Design review of the part built by this model. Coordinates are the model's own, in mm. A direction names the side the tool comes from. Give positions to 0.01 mm unless a question says otherwise; leave off trailing zeros. Loops run counter-clockwise (first coordinate to the right, second up) from the corner with the lowest first, then second, coordinate; pieces in that order, holes last. Notation, with made-up numbers: (58.5, 72) - (113.5, 72) arc R6 cw to (113.5, 78) - close; hole circle Ø8 at (49.25, -23.75). An arc over 180 degrees is marked (long way). Write each question's results on one line, items separated by ' | '.
```python
from build123d import *

# Parameters (mm, degrees)
CROQUIS1_W              = 89.98703429
CROQUIS1_H              = 59.995678097
SALIENTE_EXTRUIR1_DEPTH = 3
CROQUIS2_W              = 62
CROQUIS2_H              = 44
CORTAR_EXTRUIR1_DEPTH   = 3
CROQUIS3_W              = 5
CROQUIS3_H              = 3
SALIENTE_EXTRUIR2_DEPTH = 3
CROQUIS4_W              = 5
CROQUIS4_H              = 3
SALIENTE_EXTRUIR3_DEPTH = 3
CROQUIS5_W              = 3
CROQUIS5_H              = 5
SALIENTE_EXTRUIR4_DEPTH = 3
CROQUIS6_W              = 3
CROQUIS6_H              = 5
SALIENTE_EXTRUIR5_DEPTH = 3


with BuildPart() as part:
    # Croquis1 → Saliente-Extruir1 (new body)
    with BuildSketch(Plane.XY):
        with Locations((44.993517145, 0.761655066)):
            Rectangle(CROQUIS1_W, CROQUIS1_H)
    extrude(amount=SALIENTE_EXTRUIR1_DEPTH)

    # Croquis2 → Cortar-Extruir1 (cut)
    with BuildSketch(Plane.XY.offset(3)):
        with Locations((44.993517145, 0)):
            Rectangle(CROQUIS2_W, CROQUIS2_H)
    extrude(amount=-CORTAR_EXTRUIR1_DEPTH, mode=Mode.SUBTRACT)

    # Croquis3 → Saliente-Extruir2 (add)
    with BuildSketch(Plane(origin=(0, 30.759494114, 0), x_dir=(1, 0, 0), z_dir=(0, 1, 0))):
        with Locations((47.493517145, -1.5)):
            Rectangle(CROQUIS3_W, CROQUIS3_H)
        with Locations((42.493517145, -1.5)):
            Rectangle(CROQUIS3_W, CROQUIS3_H)
    extrude(amount=SALIENTE_EXTRUIR2_DEPTH)

    # Croquis4 → Saliente-Extruir3 (add)
    with BuildSketch(Plane.XZ.offset(29.236183983)):
        with Locations((47.493517145, 1.5)):
            Rectangle(CROQUIS4_W, CROQUIS4_H)
        with Locations((42.493517145, 1.5)):
            Rectangle(CROQUIS4_W, CROQUIS4_H)
    extrude(amount=SALIENTE_EXTRUIR3_DEPTH)

    # Croquis5 → Saliente-Extruir4 (add)
    with BuildSketch(Plane(origin=(89.98703429, 0, 0), x_dir=(0, 0, -1), z_dir=(1, 0, 0))):
        with Locations((-1.5, 3.261655066)):
            Rectangle(CROQUIS5_W, CROQUIS5_H)
        with Locations((-1.5, -1.738344934)):
            Rectangle(CROQUIS5_W, CROQUIS5_H)
    extrude(amount=SALIENTE_EXTRUIR4_DEPTH)

    # Croquis6 → Saliente-Extruir5 (add)
    with BuildSketch(Plane.ZY):
        with Locations((1.5, 3.261655066)):
            Rectangle(CROQUIS6_W, CROQUIS6_H)
        with Locations((1.5, -1.738344934)):
            Rectangle(CROQUIS6_W, CROQUIS6_H)
    extrude(amount=SALIENTE_EXTRUIR5_DEPTH)


solid = part.part
```
Item 1: Draft analysis for pull direction Y (two halves, no side actions). For faces 6 (the face through (45, -32.236, 2)), 7 (the face through (89.987, 18, 1)), 8 (the face through (75.994, 0, 2)), state which applies: +Y half, -Y half, draft (parallel to the pull), parting line (faces both ways), or undercut.
Output values:
face 6: -Y half | face 7: draft | face 8: undercut
Item 2: We need section D-D on x = 11. Give the boundary of the cut face in (y, z), then the cut area to 3 significant figures.
Output values:
outline: (-29.24, 0) - (30.76, 0) - (30.76, 3) - (-29.24, 3) - close | area: 180 mm²
Item 3: We need section A-A on y = 21. Give the boundary of the cut face in (x, z), then the cut area to 3 significant figures.
Output values:
outline: (0, 0) - (13.99, 0) - (13.99, 3) - (0, 3) - close; (75.99, 0) - (89.99, 0) - (89.99, 3) - (75.99, 3) - close | area: 84.0 mm²
Item 4: Wall thickness on probe 1 along Y at (x, z) = (34, 1.7); probe 2 along X at (y, z) = (-3, 0.9); probe 3 along X at (y, z) = (21.5, 2.85): over which ranges is each line inside the solid? List them lowest first.
Output values:
probe 1: y = -29.24 to -22, 22 to 30.76 | probe 2: x = -3 to 13.99, 75.99 to 92.99 | probe 3: x = 0 to 13.99, 75.99 to 89.99
Item 5: We need section B-B on x = 32. Give the boundary of the cut face in (y, z).
Output values:
outline: (-29.24, 0) - (-22, 0) - (-22, 3) - (-29.24, 3) - close; (22, 0) - (30.76, 0) - (30.76, 3) - (22, 3) - close
Item 6: Tool access review of faces 1 (the face through (-1, -4.238, 1)), 2 (the face through (89.987, -17, 1)), 3 (the face through (13.994, 0, 2)), 4 (the face through (49.994, 32, 2)), 5 (the face through (20, 30.759, 1)): name each direction out of +Z, -Z, +X, -X, +Y, -Y from which nothing blocks a thin tool from reaching the whole face with its end or side.
Output values:
face 1: +Z, -Z, -X, -Y | face 2: +Z, -Z, +X, -Y | face 3: +Z, -Z | face 4: +Z, -Z, +X, +Y | face 5: +Z, -Z, -X, +Y
Item 7: We need section C-C on z = 1.1. Give the boundary of the cut face in (x, y), then the cut area to 3 significant figures.
Output values:
outline: (-3, -4.24) - (0, -4.24) - (0, -29.24) - (39.99, -29.24) - (39.99, -32.24) - (49.99, -32.24) - (49.99, -29.24) - (89.99, -29.24) - (89.99, -4.24) - (92.99, -4.24) - (92.99, 5.76) - (89.99, 5.76) - (89.99, 30.76) - (49.99, 30.76) - (49.99, 33.76) - (39.99, 33.76) - (39.99, 30.76) - (0, 30.76) - (0, 5.76) - (-3, 5.76) - close; hole (13.99, -22) - (75.99, -22) - (75.99, 22) - (13.99, 22) - close | area: 2,790 mm²
Item 8: Clearance check with flat-ended pins moving along their axes: P1, Ø0.9, axis at y = -18, z = 1.5, coming from the -X side; P2, Ø1.5, axis at x = -1.5, z = 1, coming from the -Y side; P3, Ø1.5, axis at x = 92, z = 1, coming from the +Y side. State where each tip first meets the part, or that it passes through.
Output values:
P1: stops at x = 0 | P2: stops at y = -4.24 | P3: stops at y = 5.76
